Could you check a few things on this model? Use its own coordinates, in mm. A direction names the side the tool comes from. Give positions to 0.01 mm unless a question says otherwise; leave off trailing zeros. Order: outer loops, then holes, each group sorted by start corner. A loop starts at its lowest first (then second) coordinate and runs counter-clockwise, first axis right, second up. Notation, with made-up numbers: (-39.5, 70.5) -> (15.5, 70.5) arc R34 ccw to (15.5, 106.5) -> close; hole circle Ø5 at (-31.75, 28.5). An arc over 180 degrees is marked (long way). Write each question's results on one line, items separated by ' | '.
```python
from build123d import *

# Parameters (mm, degrees)
SKETCH1_R                         = 33.274
BOSS_EXTRUDE1_DEPTH               = 12.7
SKETCH2_R                         = 19.05
BOSS_EXTRUDE2_DEPTH               = 162.052
SKETCH3_R                         = 33.274
BOSS_EXTRUDE3_DEPTH               = 12.7
SKETCH4_R                         = 4.7625
BOSS_EXTRUDE4_DEPTH               = 174.752
BOSS_EXTRUDE5_START               = -0.151825
SKETCH5_R                         = 3.175
BOSS_EXTRUDE5_DEPTH               = 12.851825
BOSS_EXTRUDE6_START               = -0.151825
SKETCH6_R                         = 3.175
BOSS_EXTRUDE6_DEPTH               = 12.851825
F_1_8_NPT_TAPPED_HOLE1_AT_2_COUNT = 2
F_1_8_NPT_TAPPED_HOLE1_AT_2_PITCH = 174.752


with BuildPart() as part:
    # Sketch1 → Boss-Extrude1 (new body)
    with BuildSketch(Plane(origin=(0, 0, 0), x_dir=(0, 0, -1), z_dir=(1, 0, 0))):
        Circle(SKETCH1_R)
    extrude(amount=BOSS_EXTRUDE1_DEPTH)

    # Sketch2 → Boss-Extrude2 (add)
    with BuildSketch(Plane(origin=(12.7, 0, 0), x_dir=(0, 0, -1), z_dir=(1, 0, 0))):
        Circle(SKETCH2_R)
    extrude(amount=BOSS_EXTRUDE2_DEPTH)

    # Sketch3 → Boss-Extrude3 (add)
    with BuildSketch(Plane(origin=(174.752, 0, 0), x_dir=(0, 0, -1), z_dir=(1, 0, 0))):
        Circle(SKETCH3_R)
    extrude(amount=BOSS_EXTRUDE3_DEPTH)

    # Sketch4 → Boss-Extrude4 (add)
    with BuildSketch(Plane(origin=(187.452, 0, 0), x_dir=(0, 0, -1), z_dir=(1, 0, 0))):
        with Locations((26.4795, 0)):
            Circle(SKETCH4_R)
        with Locations((0, -26.4795)):
            Circle(SKETCH4_R)
        with Locations((-26.4795, 0)):
            Circle(SKETCH4_R)
        with Locations((0, 26.4795)):
            Circle(SKETCH4_R)
    extrude(amount=-BOSS_EXTRUDE4_DEPTH)

    # Sketch5 → Boss-Extrude5 (add)
    with BuildSketch(Plane(origin=(0, 0, -33.274), x_dir=(-1, 0, 0), z_dir=(0, 0, -1)).offset(BOSS_EXTRUDE5_START)):
        with Locations((-181.102, 0)):
            Circle(SKETCH5_R)
    extrude(amount=BOSS_EXTRUDE5_DEPTH)

    # Sketch6 → Boss-Extrude6 (add)
    with BuildSketch(Plane.XY.offset(33.274).offset(BOSS_EXTRUDE6_START)):
        with Locations((181.102, 0)):
            Circle(SKETCH6_R)
    extrude(amount=BOSS_EXTRUDE6_DEPTH)

    # Sketch8 → 1/8 NPT Tapped Hole1 (revolve, cut)
    with BuildSketch(Plane(origin=(181.102, 33.274, 0), x_dir=(0, 0, 1), z_dir=(1, 0, 0))):
        Polygon((0, 0), (0, 14.217468714), (4.2164, 11.684), (4.2164, 6.858), (4.936181096, 6.858), (5.1415188, 0), align=None)
    f_1_8_npt_tapped_hole1 = revolve(axis=Axis((181.102, 39.624, 0), (0, -1, 0)), mode=Mode.SUBTRACT)

    # 1/8 NPT Tapped Hole1 at 2: 1/8 NPT Tapped Hole1 ×2
    with Locations(*[(-i * F_1_8_NPT_TAPPED_HOLE1_AT_2_PITCH, 0, 0) for i in range(1, F_1_8_NPT_TAPPED_HOLE1_AT_2_COUNT)]):
        add(f_1_8_npt_tapped_hole1, mode=Mode.SUBTRACT)


solid = part.part
```
Q1. Suppose I cut it at B-B on y = -28.5. Please give me the cut outline in (x, z).
Here are the results:
outline: (0, -17.17) -> (12.7, -17.17) -> (12.7, -4.31) -> (174.75, -4.31) -> (174.75, -17.17) -> (187.45, -17.17) -> (187.45, 17.17) -> (174.75, 17.17) -> (174.75, 4.31) -> (12.7, 4.31) -> (12.7, 17.17) -> (0, 17.17) -> close
Q2. I need wall thicknesses on line 1 along X through (y, z) = (24, 0); line 2 along Y through (x, z) = (65, -0.5); line 3 along Y through (x, z) = (34, -3). Which ranges of each line are inside material? Lowest first, please.
Here are the results:
line 1: x = 0 to 2.13, 10.57 to 176.89, 185.32 to 187.45 | line 2: y = -31.22 to -21.74, -19.04 to 19.04, 21.74 to 31.22 | line 3: y = -30.18 to -22.78, -18.81 to 18.81, 22.78 to 30.18
Q3. For faces 1 (the cylindrical face through (178.762, 2.146, 39.458)), 2 (the flat face through (174.752, -14, -14)), 3 (the flat face through (187.452, 0, 0)), 4 (the flat face through (181, 0, -45.974)), 5 (the flat face through (179, 26.416, -4)), which set-ups out of +Z, -Z, +X, -X, +Y, -Y let a thin tool reach every point of the face, with its end or its side?
Here are the results:
face 1: +Z | face 2: none | face 3: +Z, -Z, +X, +Y, -Y | face 4: -Z, +X, -X, +Y, -Y | face 5: +Y
Q4. Suppose I cut it at A-A on x = 24.5. State how many separate pieces and enclosed holes the cut face has, and give its area (3 significant figures).
Here are the results:
separate pieces: 5 | enclosed holes: 0 | area: 1,430 mm²
Q5. Thinking about a two-plate mould opening in Z: for faces 6 (the cylindrical face through (178.17, -1.22, -39.46)), 7 (the cylindrical face through (184.84, 24.04, 1.95)), 8 (the cylindrical face through (94.86, 21.83, 1.03)), which applies, +Z half, -Z half, draft (parallel to the pull), parting line (faces both ways), or undercut?
Here are the results:
face 6: draft | face 7: undercut | face 8: parting line
Q6. Suppose I cut it at C-C on z = -28. Please give me the cut outline in (x, y).
Here are the results:
outline: (0, -17.98) -> (12.7, -17.98) -> (12.7, -4.51) -> (174.75, -4.51) -> (174.75, -17.98) -> (187.45, -17.98) -> (187.45, 17.98) -> (174.75, 17.98) -> (174.75, 4.51) -> (12.7, 4.51) -> (12.7, 17.98) -> (0, 17.98) -> close
Q7. I'm going to push flat-ended pins straight in: pin 1 Ø10 at (x, y) = (75.5, 9) entering from -Z; pin 2 Ø1.5 at (x, y) = (87.5, 14) entering from +Z; pin 3 Ø1 at (x, z) = (102.5, -26) entering from +Y. Where does each tip first touch, or does it pass through?
Here are the results:
pin 1: stops at z = -29.06 | pin 2: stops at z = 13.69 | pin 3: stops at y = 4.76
